Geometry: final body of the model. Coordinates: model frame, mm. Give positions to 0.01 mm unless a question says otherwise; leave off trailing zeros. Order: outer loops, then holes, each group sorted by start corner. A loop starts at its lowest first (then second) coordinate and runs counter-clockwise, first axis right, second up. Notation, with made-up numbers: (18.5, 2.25) - (50.5, 2.25) arc R21 cw to (50.5, 10.25) - close; hole circle Ø5 at (50.5, 21). An arc over 180 degrees is marked (long way). Put each result on its own line as item: value. Start each with the question number.
1. Section A-A on z = 2.05. Return the cut outline in (x, y).
2. Section D-D on y = 11. Return the cut outline in (x, z), plus the area to 3 significant figures.
3. Ray query, line 1 along X through (y, z) = (-2, 1.05); line 2 along Y through (x, z) = (2, 0.45); line 3 along Y through (x, z) = (-1, 0.3). Return the intervals inside material, ascending. Write a range as from..to.
4. Section B-B on y = 0. Return the cut outline in (x, z), plus the area to 3 significant figures.
5. First-contact query: P1, Ø1.5, axis at y = -8, z = 0.5, coming from the -X side. Flat tip, straight axial feed; report the tip coordinate or a pass-through.
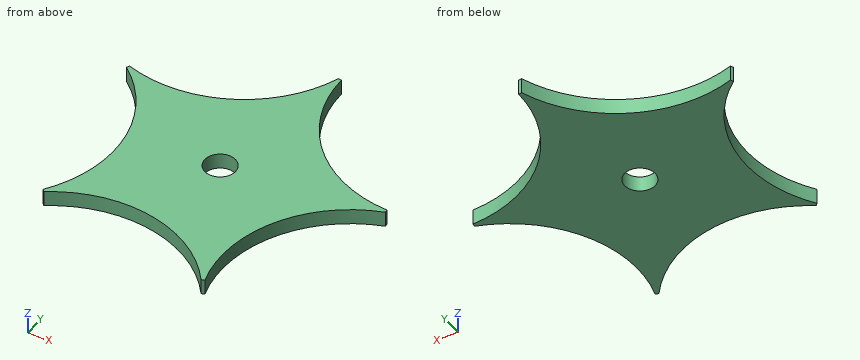
Autodesk Inventor part; units mm, degrees
ref_plane "YZ Plane" through (0, 0, 0) normal (1, 0, 0) x (0, 1, 0)
ref_plane "XZ Plane" through (0, 0, 0) normal (0, 1, 0) x (-1, 0, 0)
ref_plane "XY Plane" through (0, 0, 0) normal (0, 0, 1) x (1, 0, 0)
sketch "Sketch1" plane through (0, 0, 0) normal (0, 0, 1) x (1, 0, 0)
  circle A0 centre (0, 0) radius 30
  dimension "d0" = 60
extrude "Extrusion1" add sketch "Sketch1" along normal blind 3
sketch "Sketch2" plane through (0, 0, 3) normal (0, 0, 1) x (1, 0, 0)
  circle A0 centre (0, 0) radius 30
  circle A1 centre (30, 30) radius 25
  dimension "d6" = 50
  dimension "d7" = 30
  dimension "d8" = 30
extrude "Extrusion2" cut sketch "Sketch2" against normal through all contours A1 A0 | A0 A1 picked at (18.8229, 17.5315) picked at (30.2504, 29.5845)
pattern_circular "Circular Pattern1" count 5 over 360 about axis through (0, 0, -10) along (0, 0, 1) of "Extrusion2"
sketch "Sketch3" plane through (0, 0, 3) normal (0, 0, 1) x (1, 0, 0)
  point P0 (0, 0)
  point P1 (0, 0)
hole "Hole1" at (0, 0, 3) direction (0, 0, -1) diameter 6 end through all
properties part number "Timing_Star"
Resolved:
1. outline: (-26.87, 13.34) arc R25 cw to (-21.43, -20.99) arc R30 ccw to (-20.99, -21.43) arc R25 cw to (13.34, -26.87) arc R30 ccw to (13.9, -26.59) arc R25 cw to (29.68, 4.38) arc R30 ccw to (29.58, 5) arc R25 cw to (5, 29.58) arc R30 ccw to (4.38, 29.68) arc R25 cw to (-26.59, 13.9) arc R30 ccw to start; hole circle Ø6 at (0, 0)
2. outline: (-24.19, 0) - (13.75, 0) - (13.75, 3) - (-24.19, 3) - close
2. area: 114 mm^2
3. line 1: -17.34..-2.24, 2.24..19.72
3. line 2: -18.44..-2.24, 2.24..24.65
3. line 3: -17.55..-2.83, 2.83..20.73
4. outline: (-17.8, 0) - (-3, 0) - (-3, 3) - (-17.8, 3) - close; (3, 0) - (21.86, 0) - (21.86, 3) - (3, 3) - close
4. area: 101 mm^2
5. P1: x = -16.99
